from build123d import *

# Parameters (mm, degrees)
SKETCH1_W           = 45
SKETCH1_H           = 40
BOSS_EXTRUDE1_DEPTH = 6
CUT_EXTRUDE1_DEPTH  = 35
FILLET4_R           = 0.3
CUT_EXTRUDE4_DEPTH  = 20
CHAMFER1_SIZE       = 0.1
SKETCH10_W          = 25.487766081
SKETCH10_H          = 1.5
CUT_EXTRUDE8_DEPTH  = 47.284446632
CUT_EXTRUDE9_DEPTH  = 1.75
CUT_EXTRUDE10_DEPTH = 1.25
SKETCH13_W          = 15
SKETCH13_H          = 20
CUT_EXTRUDE11_DEPTH = 3.5
SKETCH14_W          = 15
SKETCH14_H          = 1.5
SKETCH14_W_2        = 3.5
SKETCH14_H_2        = 2
BOSS_EXTRUDE2_DEPTH = 1.5
FILLET5_R           = 1
SKETCH15_R          = 0.9
BOSS_EXTRUDE3_DEPTH = 1.5
BOSS_EXTRUDE4_START = 7
SKETCH15_3_R        = 0.9
BOSS_EXTRUDE4_DEPTH = 1
SKETCH15_4_R        = 0.9
BOSS_EXTRUDE5_DEPTH = 8
BOSS_EXTRUDE6_START = -3
BOSS_EXTRUDE6_DEPTH = 20
BOSS_EXTRUDE7_DEPTH = 2.5
BOSS_EXTRUDE8_DEPTH = 5


with BuildPart() as part:
    # Sketch1 → Boss-Extrude1 (new body)
    with BuildSketch(Plane.XY):
        Rectangle(SKETCH1_W, SKETCH1_H)
    extrude(amount=BOSS_EXTRUDE1_DEPTH)

    # Sketch2 → Cut-Extrude1 (cut)
    with BuildSketch(Plane.XZ.offset(20)):
        Polygon((-15.767949192, 6), (-14.035898385, 3), (-20.5, 3), (-18.767949192, 6), align=None)
    extrude(amount=-CUT_EXTRUDE1_DEPTH, mode=Mode.SUBTRACT)

    # Fillet4
    fillet4_edges = [part.edges().sort_by_distance(p)[0] for p in [
        (-18.767949192, -2.5, 6),
        (-15.767949192, -2.5, 6),
    ]]
    fillet(fillet4_edges, radius=FILLET4_R)

    # Sketch5 → Cut-Extrude4 (cut)
    with BuildSketch(Plane.XZ.offset(20)):
        Polygon((-9.882308546, 6), (-9.016283143, 4.5), (-12.24833395, 4.5), (-11.382308546, 6), align=None)
    extrude(amount=-CUT_EXTRUDE4_DEPTH, mode=Mode.SUBTRACT)

    # Chamfer1
    chamfer1_edges = [part.edges().sort_by_distance(p)[0] for p in [
        (-11.382308546, -10, 6),
        (-9.882308546, -10, 6),
    ]]
    chamfer(chamfer1_edges, length=CHAMFER1_SIZE)

    # Sketch10 → Cut-Extrude8 (cut, through all)
    with BuildSketch(Plane.XZ.offset(20)):
        with Locations((9.756116959, 0.75)):
            Rectangle(SKETCH10_W, SKETCH10_H)
    extrude(amount=-CUT_EXTRUDE8_DEPTH, mode=Mode.SUBTRACT)

    # Sketch11 → Cut-Extrude9 (cut, symmetric)
    with BuildSketch(Plane(origin=(-17.267949192, 0, 0), x_dir=(0, 0, -1), z_dir=(1, 0, 0))):
        Polygon((-3, -19), (-3, -6), (-2.3, -19), align=None)
    extrude(amount=CUT_EXTRUDE9_DEPTH, both=True, mode=Mode.SUBTRACT)

    # Sketch12 → Cut-Extrude10 (cut, symmetric)
    with BuildSketch(Plane(origin=(-10.632308546, 0, 0), x_dir=(0, 0, -1), z_dir=(1, 0, 0))):
        Polygon((-4.5, -19.2), (-4.5, -11.198963388), (-3.8, -19.2), align=None)
    extrude(amount=CUT_EXTRUDE10_DEPTH, both=True, mode=Mode.SUBTRACT)

    # Sketch13 → Cut-Extrude11 (cut)
    with BuildSketch(Plane.XY.offset(6)):
        with Locations((0.717691454, -7)):
            Rectangle(SKETCH13_W, SKETCH13_H)
    extrude(amount=-CUT_EXTRUDE11_DEPTH, mode=Mode.SUBTRACT)

    # Sketch14 → Boss-Extrude2 (add)
    with BuildSketch(Plane.XY.offset(6)):
        with Locations((0.717691454, -16.25)):
            Rectangle(SKETCH14_W, SKETCH14_H)
        with Locations((-5.032308546, 2)):
            Rectangle(SKETCH14_W_2, SKETCH14_H_2)
        with Locations((6.467691454, 2)):
            Rectangle(SKETCH14_W_2, SKETCH14_H_2)
    extrude(amount=-BOSS_EXTRUDE2_DEPTH)

    # Fillet5
    fillet5_edges = [part.edges().sort_by_distance(p)[0] for p in [
        (-3.282308546, 1, 5.25),
        (4.717691454, 1, 5.25),
    ]]
    fillet(fillet5_edges, radius=FILLET5_R)

    # Sketch15 → Boss-Extrude3 (add)
    # profile 1 of 2: a face of its own
    with BuildSketch(Plane(origin=(0, 0, 0), x_dir=(0, 0, -1), z_dir=(1, 0, 0))):
        with BuildLine():
            Line((2.922618262, 16.125083661), (-1.5, 14.062782897))
            Line((-1.5, 14.062782897), (-1.5, 20))
            Line((-1.5, 20), (2.922618262, 17.937699235))
            ThreePointArc((2.922618262, 17.937699235), (3.5, 17.031391448), (2.922618262, 16.125083661))
        make_face()
        with Locations((2.5, 17.031391448)):
            Circle(SKETCH15_R, mode=Mode.SUBTRACT)
    # profile 2 of 2: a face of its own
    with BuildSketch(Plane(origin=(0, 0, 0), x_dir=(0, 0, -1), z_dir=(1, 0, 0))):
        with BuildLine():
            ThreePointArc((2.922618262, -2.062300765), (3.5, -2.968608552), (2.922618262, -3.874916339))
            Line((2.922618262, -3.874916339), (-1.5, -5.937217103))
            Line((-1.5, -5.937217103), (-1.5, 0))
            Line((-1.5, 0), (2.922618262, -2.062300765))
        make_face()
        with Locations((2.5, -2.968608552)):
            Circle(SKETCH15_R, mode=Mode.SUBTRACT)
    extrude(amount=BOSS_EXTRUDE3_DEPTH)

    # Sketch15<3> → Boss-Extrude4 (add)
    # profile 1 of 2: a face of its own
    with BuildSketch(Plane(origin=(0, 0, 0), x_dir=(0, 0, -1), z_dir=(1, 0, 0)).offset(BOSS_EXTRUDE4_START)):
        with BuildLine():
            ThreePointArc((2.922618262, -2.062300765), (3.5, -2.968608552), (2.922618262, -3.874916339))
            Line((2.922618262, -3.874916339), (-1.5, -5.937217103))
            Line((-1.5, -5.937217103), (-1.5, 0))
            Line((-1.5, 0), (2.922618262, -2.062300765))
        make_face()
        with Locations((2.5, -2.968608552)):
            Circle(SKETCH15_3_R, mode=Mode.SUBTRACT)
    # profile 2 of 2: a face of its own
    with BuildSketch(Plane(origin=(0, 0, 0), x_dir=(0, 0, -1), z_dir=(1, 0, 0)).offset(BOSS_EXTRUDE4_START)):
        with BuildLine():
            Line((2.922618262, 16.125083661), (-1.5, 14.062782897))
            Line((-1.5, 14.062782897), (-1.5, 20))
            Line((-1.5, 20), (2.922618262, 17.937699235))
            ThreePointArc((2.922618262, 17.937699235), (3.5, 17.031391448), (2.922618262, 16.125083661))
        make_face()
        with Locations((2.5, 17.031391448)):
            Circle(SKETCH15_3_R, mode=Mode.SUBTRACT)
    extrude(amount=BOSS_EXTRUDE4_DEPTH)

    # Sketch15<4> → Boss-Extrude5 (add)
    with BuildSketch(Plane(origin=(0, 0, 0), x_dir=(0, 0, -1), z_dir=(1, 0, 0))):
        with Locations((2.5, 17.031391448)):
            Circle(SKETCH15_4_R)
        with Locations((2.5, -2.968608552)):
            Circle(SKETCH15_4_R)
    extrude(amount=BOSS_EXTRUDE5_DEPTH)

    # Sketch16 → Boss-Extrude6 (add)
    with BuildSketch(Plane(origin=(0, 20, 0), x_dir=(1, 0, 0), z_dir=(0, 1, 0)).offset(BOSS_EXTRUDE6_START)):
        with BuildLine():
            Line((-21, 1), (-21, 2))
            Line((-21, 2), (-18.5, 2))
            Line((-18.5, 2), (-18.5, 1))
            Line((-18.5, 1), (-20, 1))
            Line((-20, 1), (-20, 0))
            Line((-20, 0), (-22, 0))
            ThreePointArc((-22, 0), (-21.292893219, 0.292893219), (-21, 1))
        make_face()
        with BuildLine():
            Line((-5, 0), (-3, 0))
            ThreePointArc((-3, 0), (-3.707106781, 0.292893219), (-4, 1))
            Line((-4, 1), (-4, 2))
            Line((-4, 2), (-6.5, 2))
            Line((-6.5, 2), (-6.5, 1))
            Line((-6.5, 1), (-5, 1))
            Line((-5, 1), (-5, 0))
        make_face()
    extrude(amount=-BOSS_EXTRUDE6_DEPTH)

    # Sketch18 → Boss-Extrude7 (add, symmetric)
    with BuildSketch(Plane(origin=(-12.5, 0, 0), x_dir=(0, 0, 1), z_dir=(1, 0, 0))):
        with BuildLine():
            Line((-1, -19), (-2, -19))
            Line((-2, -19), (-2, -17))
            Line((-2, -17), (-1, -17))
            Line((-1, -17), (-1, -18))
            Line((-1, -18), (0, -18))
            Line((0, -18), (0, -20))
            ThreePointArc((0, -20), (-0.292893219, -19.292893219), (-1, -19))
        make_face()
    extrude(amount=BOSS_EXTRUDE7_DEPTH, both=True)

    # Sketch19 → Boss-Extrude8 (add, symmetric)
    with BuildSketch(Plane(origin=(-12.5, 0, 0), x_dir=(0, 0, -1), z_dir=(1, 0, 0))):
        with BuildLine():
            Line((0, -7.5), (1, -7.5))
            ThreePointArc((1, -7.5), (1.5, -8), (1, -8.5))
            Line((1, -8.5), (0, -8.5))
            Line((0, -8.5), (0, -7.5))
        make_face()
    extrude(amount=BOSS_EXTRUDE8_DEPTH, both=True)


solid = part.part
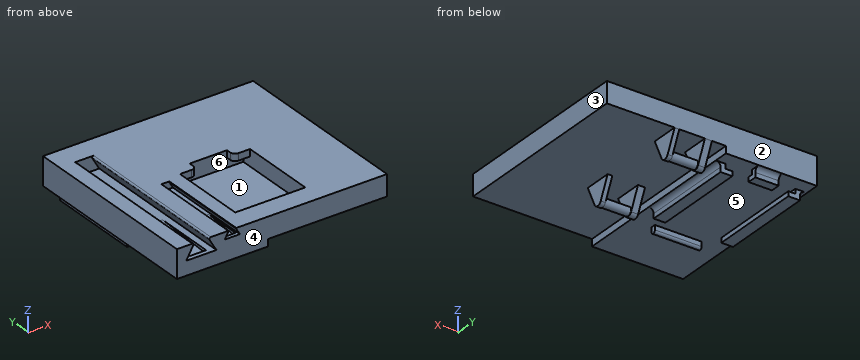
Design review of the part built by this model. Coordinates are the model's own, in mm. Face numbers are marked on the shaded views. A direction names the side the tool comes from. Give positions to 0.01 mm unless a question says otherwise; leave off trailing zeros. Write each loop counter-clockwise with the first axis right and the second up, starting at its lowest first coordinate (ties: lowest second). Pieces come first, ordered by that corner, then holes. Notation, with made-up numbers: M 19.5,69 L 31.5,69 A15 cw 31.5,97 Z; hole C 84.5,-9.5 d11. An arc over 180 degrees is marked long. Return JSON: item names as keys, results as strings. Group by question number.
Item 1: Take a section at A-A (x = 7.5). Give the boundary of the cut face in (y, z).
Item 2: Take a section at C-C (z = -0.5). Count the separate pieces of the cut face and the enclosed holes in it, plus the area to 3 significant figures.
Item 3: Clearance check with flat-ended pins moving along their axes: pin 1 Ø0.5 at (x, z) = (-11, 5) entering from -Y; pin 2 Ø2 at (x, y) = (-12.5, 17.5) entering from -Z; pin 3 Ø0.5 at (y, z) = (3, -1.5) entering from +X. State where each tip first meets the part, or that it passes through.
Item 4: Tool access review of the marked faces 1 and 2: name each direction out of +Z, -Z, +X, -X, +Y, -Y from which nothing blocks a thin tool from reaching the whole face with its end or side.
Item 5: The part is to be moulded in two halves that separate along X. For the marked faces 3, 4, 5 and 6, say which applies: pulls with the +X half, pulls with the -X half, needs draft (parallel to the pull), parting line crosses it, or undercut.
Item 6: Wall thickness on line 1 along X through (y, z) = (-5, 4.25); line 2 along Y through (x, z) = (4.5, 4); line 3 along Z through (x, y) = (-5.5, 15): over which ranges is each line inside the solid? List them lowest first.
Return value:
{
 "1": {"outline": "M -20,1.5 L -5.94,1.5 L -3.87,-2.92 A1 ccw -2.06,-2.92 L 0,1.5 L 14.06,1.5 L 16.13,-2.92 A1 ccw 17.94,-2.92 L 20,1.5 L 20,6 L 1,6 L 1,4.5 L 3,4.5 L 3,2.5 L -17,2.5 L -17,4.5 L -15.5,4.5 L -15.5,6 L -20,6 Z"},
 "2": {"separate pieces": "8", "enclosed holes": "0", "area": "81.4 mm2"},
 "3": {"pin 1": "stops at y = 0", "pin 2": "stops at z = -2", "pin 3": "stops at x = -4"},
 "4": {"face 1": "none", "face 2": "+Z, -Z, +X, -X, +Y"},
 "5": {"face 3": "pulls with the +X half", "face 4": "needs draft", "face 5": "undercut", "face 6": "undercut"},
 "6": {"line 1": "x = -22.5 to -19.78, -14.76 to -6.78, 8.22 to 22.5", "line 2": "y = -20 to -17, 3 to 20", "line 3": "z = -2 to -1, 0 to 6"}
}
